Geometry check sheet. Reference: the model listing, model coordinates, mm. Face numbers are marked on the shaded views. A direction names the side the tool comes from. Round coordinates to 2 decimals unless told otherwise and drop trailing zeros. Write each loop counter-clockwise with the first axis right and the second up, starting at its lowest first coordinate (ties: lowest second). Pieces come first, ordered by that corner, then holes.
Item 1: Access from +Z, -Z, +X, -X, +Y, -Y to the whole of each face (thin tool, end or side, straight path). Record for the marked faces 5, 6, 7 and 8.
Item 2: Scan lines: probe 1 along X at (y, z) = (6.75, 2.5); probe 2 along Y at (x, z) = (9.5, 8.25); probe 3 along Y at (x, z) = (-4.25, 2.25). Record each from-to range of solid material in increasing order.
Item 3: Depth check by flat-ended pin: P1, Ø2, axis at x = 18, z = 4.5, coming from the +Y side; P2, Ø2.5, axis at y = 5, z = 6.5, coming from the +X side; P3, Ø6.5, axis at x = -4.5, z = 5, coming from the -Y side; P4, Ø4, axis at y = 5.5, z = 4, coming from the -X side. Enter the tip coordinate at first touch or a pass-through.
Item 4: Cross-section at A-A (y = 10.5). Enter the section's corners in (x, z).
Item 5: Cross-section at B-B (y = 6.75). Enter the section's corners in (x, z), then the cut area to 3 significant figures.
Item 6: Draft check along Z on the marked faces 1, 2, 3 and 4. Enter one of: pulls with the +Z half, pulls with the -Z half, needs draft (parallel to the pull), parting line crosses it, or undercut.
Item 7: Cross-section at C-C (z = 4.5). Enter the section's corners in (x, y), then the cut area to 3 significant figures.
Item 8: Cross-section at D-D (x = -3). Enter the section's corners in (y, z) (3 decimals).
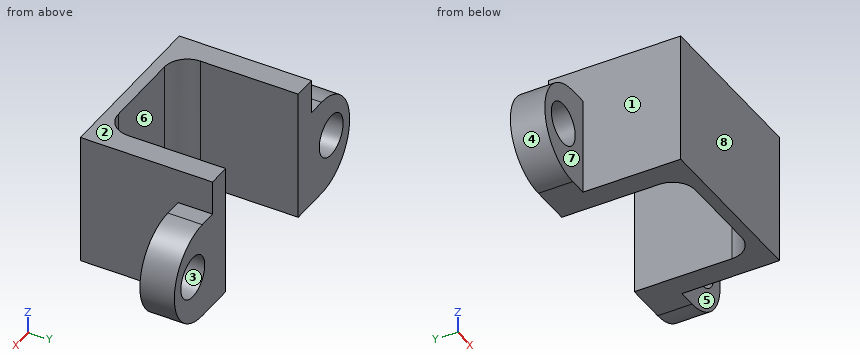
from build123d import *

# Parameters (mm, degrees)
SKETCH1_W           = 15
SKETCH1_H           = 11.5
BOSS_EXTRUDE1_DEPTH = 11.5
SKETCH3_W           = 11
SKETCH3_H           = 10.5
CUT_EXTRUDE1_DEPTH  = 11.5
FILLET1_R           = 2
BOSS_EXTRUDE2_DEPTH = 3
SKETCH5_R           = 1.809208309
CUT_EXTRUDE2_DEPTH  = 3


with BuildPart() as part:
    # Sketch1 → Boss-Extrude1 (new body)
    with BuildSketch(Plane.XY):
        with Locations((7.5, 5.75)):
            Rectangle(SKETCH1_W, SKETCH1_H)
    extrude(amount=BOSS_EXTRUDE1_DEPTH)

    # Sketch3 → Cut-Extrude1 (cut)
    with BuildSketch(Plane.XY.offset(11.5)):
        with Locations((7.5, 6.25)):
            Rectangle(SKETCH3_W, SKETCH3_H)
    extrude(amount=-CUT_EXTRUDE1_DEPTH, mode=Mode.SUBTRACT)

    # Fillet1
    fillet1_edges = [part.edges().sort_by_distance(p)[0] for p in [
        (2, 1, 5.75),
        (13, 1, 5.75),
    ]]
    fillet(fillet1_edges, radius=FILLET1_R)

    # Sketch4 → Boss-Extrude2 (add)
    with BuildSketch(Plane(origin=(0, 11.5, 0), x_dir=(1, 0, 0), z_dir=(0, 1, 0))):
        with BuildLine():
            Line((0, 0), (-1.55, 0))
            ThreePointArc((-1.55, 0), (-5.8, -4.25), (-1.55, -8.5))
            Line((-1.55, -8.5), (0, -8.5))
            Line((0, -8.5), (0, 0))
        make_face()
        with BuildLine():
            Line((15, 0), (16.55, 0))
            ThreePointArc((16.55, 0), (20.8, -4.25), (16.55, -8.5))
            Line((16.55, -8.5), (15, -8.5))
            Line((15, -8.5), (15, 0))
        make_face()
    extrude(amount=-BOSS_EXTRUDE2_DEPTH)

    # Sketch5 → Cut-Extrude2 (cut)
    with BuildSketch(Plane(origin=(0, 11.5, 0), x_dir=(1, 0, 0), z_dir=(0, 1, 0))):
        with Locations((-3, -4.5)):
            Circle(SKETCH5_R)
    cut_extrude2 = extrude(amount=-CUT_EXTRUDE2_DEPTH, mode=Mode.SUBTRACT)

    # Mirror1: Cut-Extrude2 across plane
    add(cut_extrude2.mirror(Plane.ZY.offset(-7.5)), mode=Mode.SUBTRACT)


solid = part.part
Resolved:
1. face 5: +Z, -Z, +X, -Y
1. face 6: +Z, -Z, +Y
1. face 7: +Z, -Z, -X, -Y
1. face 8: +Z, -Z, +X, -X, -Y
2. probe 1: x = 0 to 2, 13 to 15
2. probe 2: y = 0 to 1
2. probe 3: y = 8.5 to 11.5
3. P1: passes through
3. P2: stops at x = 15
3. P3: stops at y = 8.5
3. P4: stops at x = 0
4. outline: (-1.55, 0) - (2, 0) - (2, 11.5) - (0, 11.5) - (0, 8.5) - (-1.55, 8.5) arc R4.25 ccw to start; (13, 0) - (16.55, 0) arc R4.25 ccw to (16.55, 8.5) - (15, 8.5) - (15, 11.5) - (13, 11.5) - close; hole circle Ø3.62 at (-3, 4.5); hole circle Ø3.62 at (18, 4.5)
5. outline: (0, 0) - (2, 0) - (2, 11.5) - (0, 11.5) - close; (13, 0) - (15, 0) - (15, 11.5) - (13, 11.5) - close
5. area: 46.0 mm2
6. face 1: needs draft
6. face 2: pulls with the +Z half
6. face 3: undercut
6. face 4: parting line crosses it
7. outline: (-5.79, 8.5) - (-4.81, 8.5) - (-4.81, 11.5) - (-5.79, 11.5) - close; (-1.19, 8.5) - (0, 8.5) - (0, 0) - (15, 0) - (15, 8.5) - (16.19, 8.5) - (16.19, 11.5) - (13, 11.5) - (13, 3) arc R2 cw to (11, 1) - (4, 1) arc R2 cw to (2, 3) - (2, 11.5) - (-1.19, 11.5) - close; (19.81, 8.5) - (20.79, 8.5) - (20.79, 11.5) - (19.81, 11.5) - close
7. area: 71.8 mm2
8. outline: (8.5, 0.255) - (11.5, 0.255) - (11.5, 2.691) - (8.5, 2.691) - close; (8.5, 6.309) - (11.5, 6.309) - (11.5, 8.245) - (8.5, 8.245) - close
